Check sheet for the modelled part. Datum: model origin and axes. Units: mm. Face numbers are marked on the shaded views. A direction names the side the tool comes from. Round coordinates to 2 decimals unless told otherwise and drop trailing zeros. Write each loop counter-clockwise with the first axis right and the second up, starting at its lowest first coordinate (ties: lowest second). Pieces come first, ordered by that corner, then holes.
from build123d import *

# Parameters (mm, degrees)
SKETCH2_R           = 2
SKETCH2_R_2         = 3
BOSS_EXTRUDE1_DEPTH = 5


with BuildPart() as part:
    # Sketch2 → Boss-Extrude1 (new body)
    with BuildSketch(Plane.XY):
        Polygon((21, 30.75), (-24, 30.75), (-24, -26.75), (-6.5, -26.75), (-6.5, -10.75), (11.5, -10.75), (11.5, -26.75), (21, -26.75), align=None)
        with Locations((-16, -17.75)):
            Circle(SKETCH2_R, mode=Mode.SUBTRACT)
        with Locations((-18, -6.75)):
            Circle(SKETCH2_R, mode=Mode.SUBTRACT)
        with Locations((15.5, -17.75)):
            Circle(SKETCH2_R, mode=Mode.SUBTRACT)
        with Locations((13, -6.75)):
            Circle(SKETCH2_R, mode=Mode.SUBTRACT)
        with Locations((-11, 8.75)):
            Circle(SKETCH2_R_2, mode=Mode.SUBTRACT)
    extrude(amount=-BOSS_EXTRUDE1_DEPTH)


solid = part.part
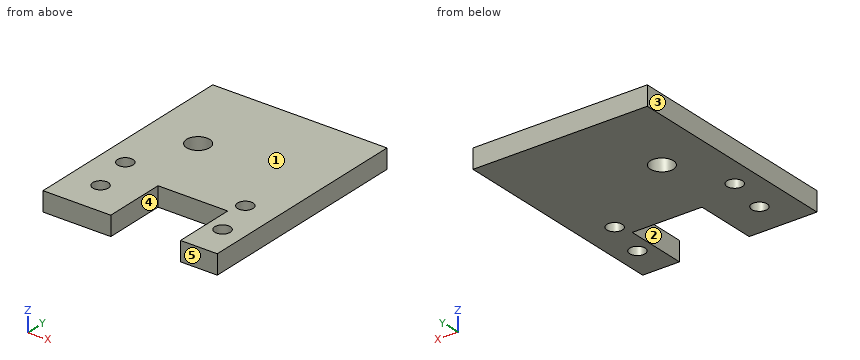
1. Sectioned sample at A-A, the plane y = -17.75. Enter the section's corners in (x, z).
2. Go/stop test with flat-tipped pins: pin 1 (5 mm diameter, centred on x = 3, y = 22.5, fed in from +Z); pin 2 (5 mm diameter, centred on x = -11, y = 8.75, fed in from -Z). Record where each tip stops, or that it passes through.
3. Release check for a two-part mould opening along X. For the marked faces 3, 4 and 5 record: released by +X, released by -X, zero draft, split by the parting line, or undercut.
4. Set-up check for the marked faces 1 and 2: record each of +Z, -Z, +X, -X, +Y, -Y from which the full face is reachable in a straight line by a thin tool's end or side.
5. Sectioned sample at B-B, the plane x = -11. Enter the section's corners in (y, z), plus the area to 4 significant figures.
6. Sectioned sample at C-C, the plane z = -4.35. Enter the section's corners in (x, y).
7. Sectioned sample at D-D, the plane y = -6.75. Enter the section's corners in (x, z), plus the area to 3 significant figures.
8. Scan lines: line 1 along Y through (x, z) = (-11, -1.8); line 2 along X through (y, z) = (-16.5, -3.1); line 3 along X through (y, z) = (-22.5, -2.45). Record each from-to range of solid material in increasing order.
Computed values:
1. outline: (-24, -5) - (-18, -5) - (-18, 0) - (-24, 0) - close; (-14, -5) - (-6.5, -5) - (-6.5, 0) - (-14, 0) - close; (11.5, -5) - (13.5, -5) - (13.5, 0) - (11.5, 0) - close; (17.5, -5) - (21, -5) - (21, 0) - (17.5, 0) - close
2. pin 1: stops at z = 0
2. pin 2: passes through
3. face 3: released by -X
3. face 4: undercut
3. face 5: zero draft
4. face 1: +Z, +X, -X, +Y, -Y
4. face 2: +Z, -Z, -Y
5. outline: (-26.75, -5) - (5.75, -5) - (5.75, 0) - (-26.75, 0) - close; (11.75, -5) - (30.75, -5) - (30.75, 0) - (11.75, 0) - close
5. area: 257.5 mm2
6. outline: (-24, -26.75) - (-6.5, -26.75) - (-6.5, -10.75) - (11.5, -10.75) - (11.5, -26.75) - (21, -26.75) - (21, 30.75) - (-24, 30.75) - close; hole circle Ø4 at (-18, -6.75); hole circle Ø4 at (-16, -17.75); hole circle Ø6 at (-11, 8.75); hole circle Ø4 at (13, -6.75); hole circle Ø4 at (15.5, -17.75)
7. outline: (-24, -5) - (-20, -5) - (-20, 0) - (-24, 0) - close; (-16, -5) - (11, -5) - (11, 0) - (-16, 0) - close; (15, -5) - (21, -5) - (21, 0) - (15, 0) - close
7. area: 185 mm2
8. line 1: y = -26.75 to 5.75, 11.75 to 30.75
8. line 2: x = -24 to -17.56, -14.44 to -6.5, 11.5 to 13.94, 17.06 to 21
8. line 3: x = -24 to -6.5, 11.5 to 21
